```python
from build123d import *

# Parameters (mm, degrees)
BOSS_EXTRUDE1_DEPTH = 10
SHELL1_T            = -5


with BuildPart() as part:
    # Sketch1 → Boss-Extrude1 (new body)
    with BuildSketch(Plane(origin=(0, 0, 0), x_dir=(1, 0, 0), z_dir=(0, 1, 0))):
        with BuildLine():
            Line((0, -15), (0, -97))
            ThreePointArc((0, -97), (-4.393398282, -107.606601718), (-15, -112))
            Line((-15, -112), (-160, -112))
            ThreePointArc((-160, -112), (-199.906147513, -104.506094408), (-234.374969534, -83.045443467))
            Line((-234.374969534, -83.045443467), (-263.846039886, -56))
            Line((-263.846039886, -56), (-234.374969534, -28.954556533))
            ThreePointArc((-234.374969534, -28.954556533), (-199.906147513, -7.493905592), (-160, 0))
            Line((-160, 0), (-15, 0))
            ThreePointArc((-15, 0), (-4.393398282, -4.393398282), (0, -15))
        make_face()
    extrude(amount=BOSS_EXTRUDE1_DEPTH)

    # Shell1
    shell1_openings = [part.faces().sort_by_distance(p)[0] for p in [
        (-116.342811862, 10, 56),
    ]]
    offset(amount=SHELL1_T, openings=shell1_openings, kind=Kind.INTERSECTION)


solid = part.part
```
Geometry check sheet. Reference: the model listing, model coordinates, mm. A direction names the side the tool comes from. Round coordinates to 2 decimals unless told otherwise and drop trailing zeros. Order: outer loops, then holes, each group sorted by start corner. A loop starts at its lowest first (then second) coordinate and runs counter-clockwise, first axis right, second up. Notation, with made-up numbers: (76, 19) - (117, 19) arc R31 cw to (117, 52) - close; hole circle Ø7 at (6, 27). An arc over 180 degrees is marked (long way). Use a Markdown table: item, result. Add a question column.
(1) Sectioned sample at B-B, the plane x = -122.5. Enter the section's corners in (y, z).
(2) Sectioned sample at C-C, the plane z = 39. Enter the section's corners in (x, y), and give its area (3 significant figures).
(3) Material ranges on line 1 along X through (y, z) = (8, 34); line 2 along Z through (x, y) = (-244.5, 7.75); line 3 along Y through (x, z) = (-41.5, 17.5), recorded low to high. Write a range as [from, to].
(4) Depth check by flat-ended pin: pin 1 (6 mm diameter, centred on x = -165, z = 55, fed in from +Y); pin 2 (1.5 mm diameter, centred on x = -186, y = 1, fed in from -Z); pin 3 (1.5 mm diameter, centred on y = 8, z = 66.5, fed in from -X); pin 4 (12 mm diameter, centred on x = -112, z = 77, fed in from -Y). Enter the tip coordinate at first touch or a pass-through.
(5) Release check for a two-part mould opening along Z. For faces 1 (the flat face through (-243.9, 7.46, 44.48)), 2 (the flat face through (-248.904, 4.93, 69.712)), 3 (the cylindrical face through (-200.438, 4.93, 7.703)) record: pulls with the +Z half, pulls with the -Z half, needs draft (parallel to the pull), parting line crosses it, or undercut.
(6) Sectioned sample at A-A, the plane y = 7.25. Enter the section's corners in (x, z), and give its area (3 significant figures).
(7) Tool access check on faces 4 (the cylindrical face through (-4.51, 4.93, 4.28)), 5 (the flat face through (-89, 7, 5)). Record the directions out of +Z, -Z, +X, -X, +Y, -Y that give a thin tool (end or side, any length) a straight path to the whole face; none if there is none.
Answers below:
| question | item | result |
|---|---|---|
| 1 | outline | (0, 0) - (10, 0) - (10, 5) - (5, 5) - (5, 107) - (10, 107) - (10, 112) - (0, 112) - close |
| 2 | outline | (-245.32, 0) - (0, 0) - (0, 10) - (-5, 10) - (-5, 5) - (-237.93, 5) - (-237.93, 10) - (-245.32, 10) - close |
| 2 | area | 1,290 mm² |
| 3 | line 1 | [-239.87, -232.48], [-5, 0] |
| 3 | line 2 | [38.25, 45.03], [66.97, 73.75] |
| 3 | line 3 | [0, 5] |
| 4 | pin 1 | y = 5 |
| 4 | pin 2 | z = 2.94 |
| 4 | pin 3 | x = -253.22 |
| 4 | pin 4 | y = 0 |
| 5 | face 1 | undercut |
| 5 | face 2 | pulls with the +Z half |
| 5 | face 3 | pulls with the -Z half |
| 6 | outline | (-263.85, 56) - (-234.37, 28.95) arc R110 ccw to (-160, 0) - (-15, 0) arc R15 ccw to (0, 15) - (0, 97) arc R15 ccw to (-15, 112) - (-160, 112) arc R110 ccw to (-234.37, 83.05) - close; hole (-256.45, 56) - (-230.99, 32.64) arc R105 ccw to (-160, 5) - (-15, 5) arc R10 ccw to (-5, 15) - (-5, 97) arc R10 ccw to (-15, 107) - (-160, 107) arc R105 ccw to (-230.99, 79.36) - close |
| 6 | area | 3,230 mm² |
| 7 | face 4 | -Z, +X, +Y, -Y |
| 7 | face 5 | +Y |
